Verification items for the finished model (mm, model axes). A direction names the side the tool comes from. Give positions to 0.01 mm unless a question says otherwise; leave off trailing zeros. Write each loop counter-clockwise with the first axis right and the second up, starting at its lowest first coordinate (ties: lowest second). Pieces come first, ordered by that corner, then holes. Notation, with made-up numbers: (6.25, 50) -> (20.25, 50) arc R13 ccw to (20.25, 74) -> close; hole circle Ø7 at (-38, -10.75). An arc over 180 degrees is marked (long way). Write item = value, one per line.
from build123d import *

# Parameters (mm, degrees)
SKETCH1_W               = 88
SKETCH1_H               = 28
BOSS_EXTRUDE1_DEPTH     = 28.2
SKETCH4_R               = 2.8
CUT_EXTRUDE1_DEPTH      = 28.2
SKETCH6_R               = 4.95
CUT_EXTRUDE2_DEPTH      = 3.2
SKETCH7_W               = 80.3
SKETCH7_H               = 20.3
CUT_EXTRUDE3_DEPTH      = 20
BOSS_EXTRUDE2_DEPTH     = 3
CHAMFER2_SIZE           = 3.4
FILLET1_R               = 2
CHAMFER3_SIZE           = 1.5
FILLET3_R               = 1.5
CHAMFER4_SIZE           = 0.75
CUT_EXTRUDE6_DEPTH      = 94.958714338
CUT_EXTRUDE6_DEPTH_BACK = 94.958714338
SKETCH11_R              = 1.65
CUT_EXTRUDE8_DEPTH      = 94.958714338
CUT_EXTRUDE8_DEPTH_BACK = 1.9
SKETCH14_R              = 3
CUT_EXTRUDE9_START      = -1.9
SKETCH15_R              = 3
CUT_EXTRUDE9_DEPTH      = 1.9


with BuildPart() as part:
    # Sketch1 → Boss-Extrude1 (new body)
    with BuildSketch(Plane(origin=(0, 0, 0), x_dir=(1, 0, 0), z_dir=(0, 1, 0))):
        Rectangle(SKETCH1_W, SKETCH1_H)
    extrude(amount=BOSS_EXTRUDE1_DEPTH)

    # Sketch4 → Cut-Extrude1 (cut)
    with BuildSketch(Plane(origin=(0, 0, 0), x_dir=(1, 0, 0), z_dir=(0, 1, 0))):
        with Locations(Location((30, 0, 0), (0, 0, 270))):
            Circle(SKETCH4_R)
        with Locations(Location((10, 0, 0), (0, 0, 270))):
            Circle(SKETCH4_R)
        with Locations(Location((-10, 0, 0), (0, 0, 270))):
            Circle(SKETCH4_R)
        with Locations(Location((-30, 0, 0), (0, 0, 270))):
            Circle(SKETCH4_R)
    extrude(amount=CUT_EXTRUDE1_DEPTH, mode=Mode.SUBTRACT)

    # Sketch6 → Cut-Extrude2 (cut)
    with BuildSketch(Plane(origin=(0, 0, 0), x_dir=(1, 0, 0), z_dir=(0, 1, 0))):
        with Locations(Location((30, 0, 0), (0, 0, 270))):
            Circle(SKETCH6_R)
        with Locations(Location((10, 0, 0), (0, 0, 270))):
            Circle(SKETCH6_R)
        with Locations(Location((-10, 0, 0), (0, 0, 270))):
            Circle(SKETCH6_R)
        with Locations(Location((-30, 0, 0), (0, 0, 270))):
            Circle(SKETCH6_R)
    extrude(amount=CUT_EXTRUDE2_DEPTH, mode=Mode.SUBTRACT)

    # Sketch7 → Cut-Extrude3 (cut)
    with BuildSketch(Plane(origin=(0, 28.2, 0), x_dir=(1, 0, 0), z_dir=(0, 1, 0))):
        Rectangle(SKETCH7_W, SKETCH7_H)
    extrude(amount=-CUT_EXTRUDE3_DEPTH, mode=Mode.SUBTRACT)

    # Sketch8 → Boss-Extrude2 (add)
    with BuildSketch(Plane.XY.offset(14)):
        with BuildLine():
            Line((-25, 24.1), (25, 24.1))
            ThreePointArc((25, 24.1), (35, 14.1), (25, 4.1))
            Line((25, 4.1), (-25, 4.1))
            ThreePointArc((-25, 4.1), (-35, 14.1), (-25, 24.1))
        make_face()
        with BuildLine():
            Line((-25, 6.1), (25, 6.1))
            ThreePointArc((25, 6.1), (33, 14.1), (25, 22.1))
            Line((25, 22.1), (-25, 22.1))
            ThreePointArc((-25, 22.1), (-33, 14.1), (-25, 6.1))
        make_face(mode=Mode.SUBTRACT)
    extrude(amount=BOSS_EXTRUDE2_DEPTH)

    # Chamfer2
    chamfer2_edges = [part.edges().sort_by_distance(p)[0] for p in [
        (-44, 14.1, -14),
        (44, 14.1, -14),
        (44, 14.1, 14),
        (-44, 14.1, 14),
    ]]
    chamfer(chamfer2_edges, length=CHAMFER2_SIZE)

    # Fillet1
    fillet1_edges = [part.edges().sort_by_distance(p)[0] for p in [
        (-35, 14.1, 14),
        (0, 4.1, 14),
        (35, 14.1, 14),
        (0, 24.1, 14),
    ]]
    fillet(fillet1_edges, radius=FILLET1_R)

    # Chamfer3
    chamfer3_edges = [part.edges().sort_by_distance(p)[0] for p in [
        (0, 0, 14),
        (0, 28.2, 14),
        (-44, 0, 0),
        (0, 0, -14),
        (44, 0, 0),
        (-42.3, 0, -12.3),
        (42.3, 0, -12.3),
        (42.3, 0, 12.3),
        (-42.3, 0, 12.3),
        (-44, 28.2, 0),
        (44, 28.2, 0),
        (0, 28.2, -14),
        (-42.3, 28.2, -12.3),
        (42.3, 28.2, -12.3),
        (42.3, 28.2, 12.3),
        (-42.3, 28.2, 12.3),
    ]]
    chamfer(chamfer3_edges, length=CHAMFER3_SIZE)

    # Fillet3
    # the kernel refuses this fillet: 1.5 mm, written as the material it takes off along each edge
    with BuildSketch(Plane(origin=(44, -0.053300859, -10.6), x_dir=(0, 0, 1), z_dir=(0, 1, 0)), Plane(origin=(40.6, -0.053300859, -14), x_dir=(0.7071067811865476, 0, 0.7071067811865476), z_dir=(0, 1, 0)), Plane(origin=(44, -0.053300859, 10.6), x_dir=(-0.707106781186546, 0, 0.7071067811865489), z_dir=(0, 1, 0)), Plane(origin=(40.6, -0.053300859, 14), x_dir=(-1, 0, 0), z_dir=(0, 1, 0))) as fillet3_piece_1:
        with BuildLine():
            CenterArc((FILLET3_R * 0.414213562373, -FILLET3_R), FILLET3_R, 90, 45)
            Line((-FILLET3_R * 0.292893218813, -FILLET3_R * 0.292893218813), (0, 0))
            Line((0, 0), (FILLET3_R * 0.414213562373, 0))
        make_face()
    extrude(amount=28.306601718, mode=Mode.SUBTRACT)
    with BuildSketch(Plane(origin=(-40.6, -0.053300859, 14), x_dir=(1, 0, 0), z_dir=(0, 1, 0)), Plane(origin=(-44, -0.053300859, 10.6), x_dir=(0.7071067811865476, 0, 0.7071067811865476), z_dir=(0, 1, 0)), Plane(origin=(-44, -0.053300859, -10.6), x_dir=(0, 0, 1), z_dir=(0, 1, 0)), Plane(origin=(-40.6, -0.053300859, -14), x_dir=(-0.7071067811865476, 0, 0.7071067811865476), z_dir=(0, 1, 0))) as fillet3_piece_2:
        with BuildLine():
            CenterArc((FILLET3_R * 0.414213562373, FILLET3_R), FILLET3_R, 225, 45)
            Line((-FILLET3_R * 0.292893218813, FILLET3_R * 0.292893218813), (0, 0))
            Line((0, 0), (FILLET3_R * 0.414213562373, 0))
        make_face()
    extrude(amount=28.306601718, mode=Mode.SUBTRACT)
    with BuildSketch(Plane(origin=(-40.896282151, 25.984711613, 14.715288387), x_dir=(0.9596829822606673, -0.19875685341551574, 0.19875685341551153), z_dir=(0.2810846377148206, 0.678598344545847, -0.678598344545847)), Plane(origin=(41.784711613, 28.915288387, -9.682397506), x_dir=(0.19875685341552204, -0.1987568534155052, 0.9596829822606672), z_dir=(0.678598344545847, -0.678598344545847, -0.2810846377148206)), Plane(origin=(39.682397506, 28.915288387, -11.784711613), x_dir=(0.8191406634032525, -0.19875685341551952, 0.5380560256884418), z_dir=(0.2810846377148208, -0.678598344545847, -0.678598344545847)), Plane(origin=(-41.784711613, -0.715288387, -9.682397506), x_dir=(-0.1987568534155126, 0.19875685341551472, 0.9596829822606672), z_dir=(-0.678598344545847, 0.678598344545847, -0.2810846377148206)), Plane(origin=(40.896282151, 2.215288387, 14.715288387), x_dir=(-0.9596829822606671, 0.1987568534155152, 0.19875685341551202), z_dir=(-0.2810846377148206, -0.678598344545847, -0.678598344545847)), Plane(origin=(-39.682397506, -0.715288387, -11.784711613), x_dir=(-0.8191406634032554, 0.19875685341551527, 0.5380560256884387), z_dir=(-0.2810846377148208, 0.678598344545847, -0.678598344545847))) as fillet3_piece_3:
        with BuildLine():
            CenterArc((FILLET3_R * 0.281084637715, FILLET3_R), FILLET3_R, 238.60028519, 31.39971481)
            Line((-FILLET3_R * 0.239920745565, FILLET3_R * 0.146446609407), (0, 0))
            Line((0, 0), (FILLET3_R * 0.281084637715, 0))
        make_face()
    extrude(amount=4.31857342, mode=Mode.SUBTRACT)
    with BuildSketch(Plane(origin=(-41.784711613, 28.915288387, 9.682397506), x_dir=(0.5380560256884337, -0.19875685341550817, 0.8191406634032606), z_dir=(-0.678598344545847, -0.678598344545847, 0.2810846377148207)), Plane(origin=(-41.784711613, 28.915288387, -9.682397506), x_dir=(-0.1987568534155052, -0.19875685341552204, 0.9596829822606672), z_dir=(-0.678598344545847, -0.678598344545847, -0.2810846377148206)), Plane(origin=(-40.896282151, 2.215288387, 14.715288387), x_dir=(0.9596829822606672, 0.1987568534155143, 0.19875685341551325), z_dir=(0.2810846377148208, -0.678598344545847, -0.678598344545847)), Plane(origin=(41.784711613, -0.715288387, 9.682397506), x_dir=(-0.5380560256884355, 0.19875685341551075, 0.8191406634032589), z_dir=(0.678598344545847, 0.678598344545847, 0.2810846377148207)), Plane(origin=(39.682397506, -0.715288387, -11.784711613), x_dir=(0.819140663403258, 0.1987568534155118, 0.5380560256884362), z_dir=(0.2810846377148208, 0.678598344545847, -0.678598344545847)), Plane(origin=(41.784711613, -0.715288387, -9.682397506), x_dir=(0.1987568534155142, 0.19875685341551314, 0.9596829822606673), z_dir=(0.678598344545847, 0.678598344545847, -0.2810846377148206))) as fillet3_piece_4:
        with BuildLine():
            CenterArc((FILLET3_R * 0.281084637715, -FILLET3_R), FILLET3_R, 90, 31.39971481)
            Line((-FILLET3_R * 0.239920745565, -FILLET3_R * 0.146446609407), (0, 0))
            Line((0, 0), (FILLET3_R * 0.281084637715, 0))
        make_face()
    extrude(amount=4.31857342, mode=Mode.SUBTRACT)

    # Chamfer4
    chamfer4_edges = [part.edges().sort_by_distance(p)[0] for p in [
        (30, 0, -4.95),
        (10, 0, -4.95),
        (-10, 0, -4.95),
        (-30, 0, -4.95),
    ]]
    chamfer(chamfer4_edges, length=CHAMFER4_SIZE)

    # Sketch11 → Cut-Extrude6 (cut, two sides: drawn at the far end of the back side and taken through both)
    with BuildSketch(Plane(origin=(44, 0, 0), x_dir=(0, 0, -1), z_dir=(1, 0, 0)).offset(-CUT_EXTRUDE6_DEPTH_BACK)):
        with Locations((0, 14.1)):
            Circle(SKETCH11_R)
    extrude(amount=CUT_EXTRUDE6_DEPTH + CUT_EXTRUDE6_DEPTH_BACK, mode=Mode.SUBTRACT)

    # Sketch14 → Cut-Extrude8 (cut, two sides: drawn at the far end of the back side and taken through both)
    with BuildSketch(Plane(origin=(44, 0, 0), x_dir=(0, 0, -1), z_dir=(1, 0, 0)).offset(-CUT_EXTRUDE8_DEPTH_BACK)):
        with Locations(Location((0, 14.1, 0), (0, 0, 180))):
            Circle(SKETCH14_R)
    extrude(amount=CUT_EXTRUDE8_DEPTH + CUT_EXTRUDE8_DEPTH_BACK, mode=Mode.SUBTRACT)

    # Sketch15 → Cut-Extrude9 (cut)
    with BuildSketch(Plane.ZY.offset(44).offset(CUT_EXTRUDE9_START)):
        with Locations((0, 14.1)):
            Circle(SKETCH15_R)
    extrude(amount=CUT_EXTRUDE9_DEPTH, mode=Mode.SUBTRACT)


solid = part.part
Item 1: Sectioned sample at D-D on z = 0.5. Give the number of separate pieces and of enclosed holes in the cut face, then the cut area to 3 significant figures.
Response values:
separate_pieces = 7
enclosed_holes = 0
area = 598 mm^2
Item 2: Sectioned sample at C-C on x = -21. Record the cut outline in (y, z).
Response values:
outline = (0, -12.5) -> (1.5, -14) -> (26.7, -14) -> (28.2, -12.5) -> (28.2, -10.15) -> (8.2, -10.15) -> (8.2, 10.15) -> (28.2, 10.15) -> (28.2, 12.5) -> (26.7, 14) -> (26.1, 14) arc R2 cw to (24.1, 16) -> (24.1, 17) -> (22.1, 17) -> (22.1, 14) -> (6.1, 14) -> (6.1, 17) -> (4.1, 17) -> (4.1, 16) arc R2 cw to (2.1, 14) -> (1.5, 14) -> (0, 12.5) -> close
Item 3: Set-up check for faces 4 (the flat face through (27.9, 3.2, 2.1)), 5 (the flat face through (41.758, 0.761, 11.797)), 6 (the flat face through (-0.2, 1.9, 14)), 7 (the cylindrical face through (-43.037, 17.074, -0.391)): record each of +Z, -Z, +X, -X, +Y, -Y from which the full face is reachable in a straight line by a thin tool's end or side.
Response values:
face_4 = -Y
face_5 = +Z, +X, -Y
face_6 = +Z
face_7 = -X
Item 4: Mould release check, pull along X, two halves, no side actions. Record for faces 1 (the cylindrical face through (12.36, 5.66, 1.51)), 2 (the flat face through (0.2, 22.3, 17)), 3 (the cylindrical face through (-43.126, 27.497, -10.232)): +X half, -X half, draft (parallel to the pull), parting line (faces both ways), or undercut.
Response values:
face_1 = undercut
face_2 = draft
face_3 = -X half
Item 5: Go/stop test with flat-tipped pins: P1, Ø6.5, axis at x = -10, z = 0, coming from the +Y side; P2, Ø3, axis at x = -28, z = 0, coming from the -Y side; P3, Ø4.5, axis at x = 30, z = 0, coming from the +Y side; P4, Ø4.5, axis at y = 14.1, z = 0, coming from the +X side. Record where each tip stops, or that it passes through.
Response values:
P1 = 8.2
P2 = 3.2
P3 = through
P4 = 42.1
Item 6: Sectioned sample at B-B on z = 8. Record the cut outline in (x, y), then the cut area to 3 significant figures.
Response values:
outline = (-44, 1.5) -> (-42.5, 0) -> (42.5, 0) -> (44, 1.5) -> (44, 26.7) -> (42.5, 28.2) -> (40.15, 28.2) -> (40.15, 8.2) -> (-40.15, 8.2) -> (-40.15, 28.2) -> (-42.5, 28.2) -> (-44, 26.7) -> close
area = 871 mm^2
Item 7: Material ranges on line 1 (X direction, y = 5.85, z = 0); line 2 (X direction, y = 2.5, z = 0); line 3 (X direction, y = 9.75, z = -7.5), recorded low to high.
Response values:
line_1 = -44 to -32.8, -27.2 to -12.8, -7.2 to 7.2, 12.8 to 27.2, 32.8 to 44
line_2 = -44 to -34.95, -25.05 to -14.95, -5.05 to 5.05, 14.95 to 25.05, 34.95 to 44
line_3 = -44 to -40.15, 40.15 to 44
